Build history of the part. All positions in model axes, mm. Face numbers are marked on the shaded views. A direction names the side the tool comes from. Give positions to 0.01 mm unless a question says otherwise; leave off trailing zeros. Write each loop counter-clockwise with the first axis right and the second up, starting at its lowest first coordinate (ties: lowest second). Pieces come first, ordered by that corner, then holes. Notation, with made-up numbers: (30.25, 33.5) -> (75.25, 33.5) arc R27 ccw to (75.25, 52.5) -> close; hole circle Ø7 at (-10.5, 78). An arc over 180 degrees is marked (long way). Write item = value, one per line. Start each with the question number.
Q1. Saw through at C-C, the plane y = 3.5. List the corners of the cut face in (x, z), then the cut area to 3 significant figures.
Q2. Saw through at A-A, the plane x = 26. List the corners of the cut face in (y, z), then the cut area to 3 significant figures.
Q3. Tool access for the marked faces 1, 2 and 3: list every direction of +Z, -Z, +X, -X, +Y, -Y with a clear straight run to the whole face (end or side of a thin tool).
Q4. Drop a flat-ended pin along its axis: P1, Ø1.2, axis at y = 15, z = 2.5, coming from the -X side. Give the stop position or say it passes through.
Q5. Wall check: line 1 (Y direction, x = 19, z = 1.65); line 2 (Y direction, x = 23, z = 0.7); line 3 (X direction, y = 8.5, z = 2.1). Give the ranges that are in metal, low to high.
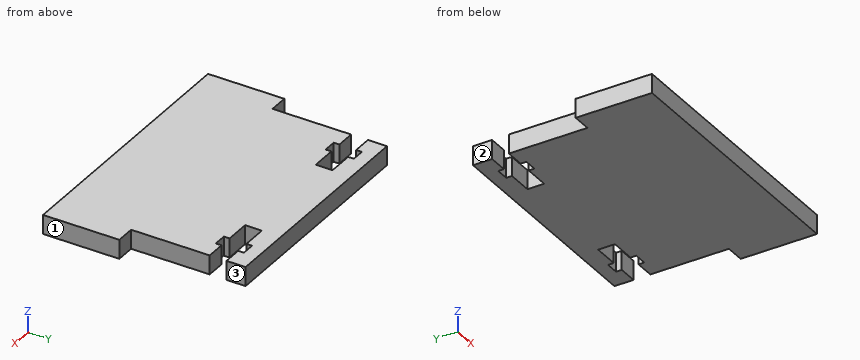
from build123d import *

# Parameters (mm, degrees)
SKETCH1_W           = 60
SKETCH1_H           = 50
BOSS_EXTRUDE1_DEPTH = 5
CUT_EXTRUDE1_DEPTH  = 5
SKETCH6_W           = 5
SKETCH6_H           = 20
BOSS_EXTRUDE2_DEPTH = 5


with BuildPart() as part:
    # Sketch1 → Boss-Extrude1 (new body)
    with BuildSketch(Plane.XY):
        Rectangle(SKETCH1_W, SKETCH1_H)
    extrude(amount=BOSS_EXTRUDE1_DEPTH)

    # Sketch5 → Cut-Extrude1 (cut)
    with BuildSketch(Plane.XY.offset(5)):
        Polygon((-30, 15.6), (-30, 20), (-25, 20), (-25, 21.5), (-21.6, 21.5), (-21.6, 20), (-15, 20), (-15, 15.6), (-21.6, 15.6), (-21.6, 14.1), (-25, 14.1), (-25, 15.6), align=None)
        Polygon((30, 20), (25, 20), (25, 21.5), (21.6, 21.5), (21.6, 20), (15, 20), (15, 15.6), (21.6, 15.6), (21.6, 14.1), (25, 14.1), (25, 15.6), (30, 15.6), align=None)
    extrude(amount=-CUT_EXTRUDE1_DEPTH, mode=Mode.SUBTRACT)

    # Sketch6 → Boss-Extrude2 (add)
    with BuildSketch(Plane(origin=(0, 0, 0), x_dir=(-1, 0, 0), z_dir=(0, 0, -1))):
        with Locations((-32.5, -15)):
            Rectangle(SKETCH6_W, SKETCH6_H)
        with Locations((32.5, -15)):
            Rectangle(SKETCH6_W, SKETCH6_H)
    extrude(amount=-BOSS_EXTRUDE2_DEPTH)


solid = part.part
Report:
q1.outline = (-30, 0) -> (30, 0) -> (30, 5) -> (-30, 5) -> close
q1.area = 300 mm2
q2.outline = (-25, 0) -> (15.6, 0) -> (15.6, 5) -> (-25, 5) -> close; (20, 0) -> (25, 0) -> (25, 5) -> (20, 5) -> close
q2.area = 228 mm2
q3.face_1 = +Z, -Z, +X, +Y, -Y
q3.face_2 = +Z, -Z, -X, +Y
q3.face_3 = +Z, -Z, +X, +Y
q4.P1 = -30
q5.line_1 = -25 to 15.6, 20 to 25
q5.line_2 = -25 to 14.1, 21.5 to 25
q5.line_3 = -30 to 30
